Check sheet for the drawn part. Datum: minimum x, y, z corner. Units: mm. A direction names the side the tool comes from. Coordinates: 2 decimals unless noted, no trailing zeros. Order: outer loops, then holes, each group sorted by start corner. A loop starts at its lowest first (then second) coordinate and runs counter-clockwise, first axis right, second up. Notation, with made-up numbers: (-36.75, 79) - (-30.75, 79) arc R34 ccw to (-30.75, 111) - close; hole circle Ø1 at (37.25, 3). An arc over 180 degrees is marked (long way). One line per item, written item: value. Start each with the question number.
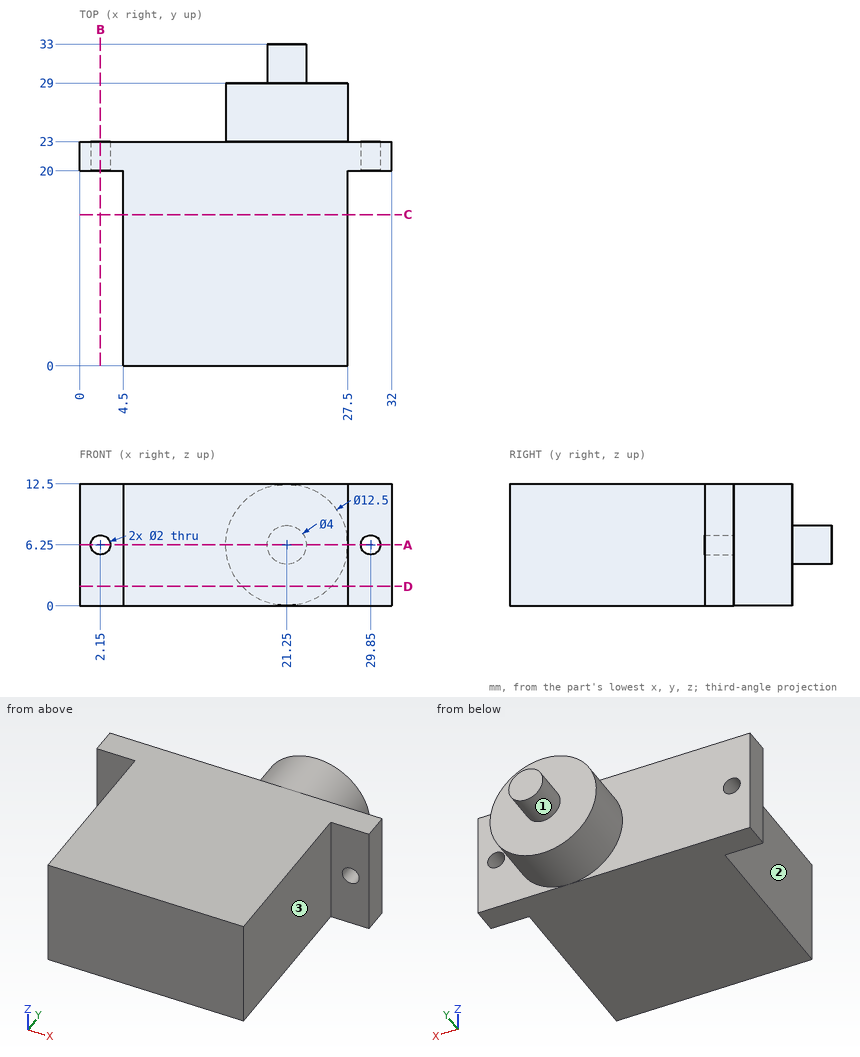
Q1. Set-up check for the marked faces 1, 2 and 3: record each of +Z, -Z, +X, -X, +Y, -Y from which the full face is reachable in a straight line by a thin tool's end or side.
Q2. Cross-section at B-B, the plane x = 2.15. Enter the section's corners in (y, z), and give its area (3 significant figures).
Q3. Cross-section at A-A, the plane z = 6.25. Enter the section's corners in (x, y), and give its area (3 significant figures).
Q4. Material ranges on probe 1 along X at (y, z) = (20.8, 6.25); probe 2 along Y at (x, z) = (23.5, 9.5); probe 3 along Y at (x, z) = (2, 1.75), recorded low to high.
Q5. Cross-section at C-C, the plane y = 15.5. Enter the section's corners in (x, z), and give its area (4 significant figures).
Q6. Cross-section at D-D, the plane z = 2. Enter the section's corners in (x, y), and give its area (3 significant figures).
Q7. Gauge pin test, flat ends, axial feed: P1, Ø1.5, axis at x = 12.5, z = 9.5, coming from the +Y side; P2, Ø5, axis at y = 7, z = 5, coming from the +X side; P3, Ø2, axis at x = 3, z = 3.5, coming from the -Y side; P4, Ø1.6, axis at x = 29.85, z = 6.25, coming from the +Y side. Record the tip position at first contact, or that the pin passes through.
Check result:
1. face 1: +Y
1. face 2: +Z, -Z, -X, -Y
1. face 3: +Z, -Z, +X, -Y
2. outline: (20, 0) - (23, 0) - (23, 5.25) - (20, 5.25) - close; (20, 7.25) - (23, 7.25) - (23, 12.5) - (20, 12.5) - close
2. area: 31.5 mm2
3. outline: (0, 20) - (1.15, 20) - (1.15, 23) - (0, 23) - close; (3.15, 20) - (4.5, 20) - (4.5, 0) - (27.5, 0) - (27.5, 20) - (28.85, 20) - (28.85, 23) - (27.5, 23) - (27.5, 29) - (23.25, 29) - (23.25, 33) - (19.25, 33) - (19.25, 29) - (15, 29) - (15, 23) - (3.15, 23) - close; (30.85, 20) - (32, 20) - (32, 23) - (30.85, 23) - close
3. area: 635 mm2
4. probe 1: x = 0 to 1.15, 3.15 to 28.85, 30.85 to 32
4. probe 2: y = 0 to 29
4. probe 3: y = 20 to 23
5. outline: (4.5, 0) - (27.5, 0) - (27.5, 12.5) - (4.5, 12.5) - close
5. area: 287.5 mm2
6. outline: (0, 20) - (4.5, 20) - (4.5, 0) - (27.5, 0) - (27.5, 20) - (32, 20) - (32, 23) - (25.83, 23) - (25.83, 29) - (16.67, 29) - (16.67, 23) - (0, 23) - close
6. area: 611 mm2
7. P1: stops at y = 23
7. P2: stops at x = 27.5
7. P3: stops at y = 20
7. P4: passes through
